Design review of the part built by this model. Coordinates are the model's own, in mm. Face numbers are marked on the shaded views. A direction names the side the tool comes from. Coordinates: 2 decimals unless noted, no trailing zeros. Order: outer loops, then holes, each group sorted by start corner. A loop starts at its lowest first (then second) coordinate and runs counter-clockwise, first axis right, second up. Notation, with made-up numbers: M 21.25,77 L 47.25,77 A11 ccw 47.25,97 Z; hole C 86,31 d9. An arc over 180 degrees is marked long. Answer as a JSON object with one key per item and string values.
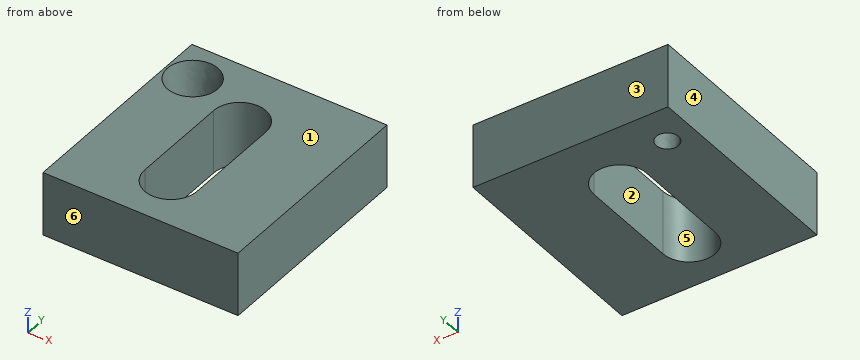
from build123d import *

# Parameters (mm, degrees)
SKETCH1_W           = 38.742575614
SKETCH1_H           = 42.674371655
BOSS_EXTRUDE1_DEPTH = 12.7


with BuildPart() as part:
    # Sketch1 → Boss-Extrude1 (new body)
    with BuildSketch(Plane.XY):
        with Locations((5.370258006, 21.337185828)):
            Rectangle(SKETCH1_W, SKETCH1_H)
        with BuildLine():
            Line((9.589746439, 29.824111426), (9.589746439, 10.069233761))
            ThreePointArc((9.589746439, 10.069233761), (4.411283362, 4.890770684), (-0.767179715, 10.069233761))
            Line((-0.767179715, 10.069233761), (-0.767179715, 29.824111426))
            ThreePointArc((-0.767179715, 29.824111426), (4.411283362, 35.002574503), (9.589746439, 29.824111426))
        make_face(mode=Mode.SUBTRACT)
    extrude(amount=BOSS_EXTRUDE1_DEPTH)

    # Cut-Loft1: read off the stored shape, not the designer's step
    # Cut-Loft1: loft between two sections, ruled curve by curve
    cut_loft1_from = [
        Edge.make_bspline([(-6.388735864, 35.417554769, 0), (-7.120249807, 39.787035762, 0), (-11.489730799, 39.055521819, 0), (-10.758216856, 34.686040826, 0), (-10.026702913, 30.316559834, 0), (-5.657221921, 31.048073777, 0), (-6.388735864, 35.417554769, 0)], [0, 0, 0, 0, 0.5, 0.5, 0.5, 1, 1, 1, 1], 3, [1, 0.333333333, 0.333333333, 1, 0.333333333, 0.333333333, 1]),
    ]
    cut_loft1_to = [
        Edge.make_bspline([(-4.568610902, 38.062672565, 12.7), (-10.590360438, 46.072403481, 12.7), (-18.600091353, 40.050653945, 12.7), (-12.578341818, 32.04092303, 12.7), (-6.556592282, 24.031192114, 12.7), (1.453138633, 30.05294165, 12.7), (-4.568610902, 38.062672565, 12.7)], [0, 0, 0, 0, 0.5, 0.5, 0.5, 1, 1, 1, 1], 3, [1, 0.333333333, 0.333333333, 1, 0.333333333, 0.333333333, 1]),
    ]
    cut_loft1 = Solid(Shell([*[Face.make_surface_from_curves(cut_loft1_from[k], cut_loft1_to[k]) for k in range(1)], Face(Wire(cut_loft1_from)), Face(Wire(cut_loft1_to))]))
    add(cut_loft1, mode=Mode.SUBTRACT)


solid = part.part
1) Tool access review of the marked faces 1 and 2: name each direction out of +Z, -Z, +X, -X, +Y, -Y from which nothing blocks a thin tool from reaching the whole face with its end or side.
Taken from the geometry:
{"face 1": "+Z, +X, -X, +Y, -Y", "face 2": "+Z, -Z"}
2) Insertion check: pin 1 Ø5 at (x, y) = (5, 28.5) entering from -Z (3 decimals). The pin has a flat end and moves straight along its axis. Give the tip position at first contact, or say it passes through.
Taken from the geometry:
{"pin 1": "passes through"}
3) To check wall thickness, follow L1, parallel to X at y = 29, z = 1.5; L2, parallel to Y at x = 6.5, z = 1.25; L3, parallel to Y at x = 2, z = 8. State the ranges of each line that lie inside material, in increasing order.
Taken from the geometry:
{"L1": "x = -14 to -0.77, 9.59 to 24.74", "L2": "y = 0 to 5.33, 34.56 to 42.67", "L3": "y = 0 to 5.49, 34.41 to 42.67"}
4) Add section B-B (x = 6.5). State the section outline as (y, z) points.
Taken from the geometry:
{"outline": "M 0,0 L 5.33,0 L 5.33,12.7 L 0,12.7 Z; M 34.56,0 L 42.67,0 L 42.67,12.7 L 34.56,12.7 Z"}
5) Add section A-A (y = 23). State the section outline as (x, z) points, and give its area (3 significant figures).
Taken from the geometry:
{"outline": "M -14,0 L -0.77,0 L -0.77,12.7 L -14,12.7 Z; M 9.59,0 L 24.74,0 L 24.74,12.7 L 9.59,12.7 Z", "area": "360 mm2"}
6) Mouldability with a two-part tool opening along Y and no side actions: class the marked faces 3, 4, 5 and 6 as released by +Y, released by -Y, zero draft, split by the parting line, or undercut.
Taken from the geometry:
{"face 3": "released by +Y", "face 4": "zero draft", "face 5": "undercut", "face 6": "released by -Y"}
7) Add section C-C (y = 33.5). Count the separate pieces of the cut face and the enclosed holes in it, and give its area (3 significant figures).
Taken from the geometry:
{"separate pieces": "3", "enclosed holes": "0", "area": "319 mm2"}
